Autodesk Inventor part; units mm, degrees
ref_plane "Work Plane8" through (0, 0, 0) normal (0, 0, -1) x (-0.8661856, 0.4997225, 0)
ref_plane "YZ Plane" through (0, 0, 0) normal (1, 0, 0) x (0, 1, 0)
ref_plane "XZ Plane" through (0, 0, 0) normal (0, 1, 0) x (-1, 0, 0)
sketch "Sketch1" plane through (0, 0, 0) normal (0, 0, 1) x (1, 0, 0)
  circle A0 centre (0, 0) radius 14.2875
  circle A1 centre (0, 0) radius 17.4625
  circle A2 centre (0, 0) radius 19.05
  dimension "d0" = 28.575
  dimension "d1" = 34.925
  dimension "d2" = 38.1
extrude "Extrusion1" add sketch "Sketch1" along normal blind 38.1 contours A0 | A1 | A2
sketch "Sketch11" plane through (0, 0, 0) normal (0, 0, 1) x (1, 0, 0)
  circle A0 centre (0, 0) radius 25.908
  circle A1 centre (-38.1, -66.04) radius 12.7
  circle A2 centre (-38.1, -66.04) radius 14.732
  circle A3 centre (-38.1, -66.04) radius 15.748
  line L0 (-38.1, -66.04) -> (-49.1429, -85.181)
  line L1 (-38.1, -66.04) -> (0, 0)
  line L2 (-38.1, -66.04) -> (-49.1551, -46.9061)
  line L3 (-38.1, -66.04) -> (-16.002, -66.0329)
  circle A4 centre (-49.1429, -85.181) radius 1.9844
  circle A5 centre (-49.1551, -46.9061) radius 1.9844
  circle A6 centre (-16.002, -66.0329) radius 1.9844
  circle A7 centre (-16.002, -66.0329) radius 5.5563
  circle A8 centre (-49.1429, -85.181) radius 5.5563
  circle A9 centre (-49.1551, -46.9061) radius 5.5563
  line L4 (-54.6991, -85.1827) -> (-54.7114, -46.9079)
  line L5 (-46.3632, -89.9919) -> (-13.2223, -70.8439)
  line L6 (-13.2254, -61.2202) -> (-46.3785, -42.0934)
  line L7 (0, 0) -> (0, -25.908)
  circle A10 centre (16.002, -66.0329) radius 1.9844
  circle A11 centre (49.1551, -46.9061) radius 1.9844
  circle A12 centre (49.1429, -85.181) radius 1.9844
  line L8 (0, 0) -> (-41.3682, 23.8663)
  line L9 (0, 0) -> (24.0327, 41.6566)
  line L10 (0, 0) -> (61.3648, -35.4028)
  dimension "d137" = 51.816
  dimension "d154" = 0
  dimension "d155" = 360
  dimension "d138" = 38.1
  dimension "d139" = 66.04
  dimension "d140" = 25.4
  dimension "d141" = 29.464
  dimension "d142" = 31.496
  dimension "d143" = 22.098
  dimension "d144" = 120
  dimension "d145" = 120
  dimension "d146" = 22.098
  dimension "d147" = 22.098
  dimension "d148" = 3.9688
  dimension "d149" = 3.9688
  dimension "d150" = 3.9688
  dimension "d151" = 11.1125
  dimension "d152" = 11.1125
  dimension "d153" = 11.1125
  dimension "d159" = 90
  dimension "d160" = 90
  dimension "d161" = 180
ref_plane "Work Plane8" through (0, 0, 0) normal (0, 0, -1) x (-0.8661856, 0.4997225, 0)
sketch "Sketch12" plane through (0, 0, 0) normal (0, 0, -1) x (-0.8661856, 0.4997225, 0)
  circle A0 centre (0, 0) radius 25.908
  circle A1 centre (-38.1, -66.04) radius 12.7
  circle A2 centre (-38.1, -66.04) radius 14.732
  circle A3 centre (-38.1, -66.04) radius 15.748
  line L0 (-38.1, -66.04) -> (-49.1429, -85.181)
  line L1 (-38.1, -66.04) -> (0, 0)
  line L2 (-38.1, -66.04) -> (-49.1551, -46.9061)
  line L3 (-38.1, -66.04) -> (-16.002, -66.0329)
  circle A4 centre (-49.1429, -85.181) radius 1.9844
  circle A5 centre (-49.1551, -46.9061) radius 1.9844
  circle A6 centre (-16.002, -66.0329) radius 1.9844
  circle A7 centre (-16.002, -66.0329) radius 5.5563
  circle A8 centre (-49.1429, -85.181) radius 5.5563
  circle A9 centre (-49.1551, -46.9061) radius 5.5563
  line L4 (-54.6991, -85.1827) -> (-54.7114, -46.9079)
  line L5 (-46.3632, -89.9919) -> (-13.2223, -70.8439)
  line L6 (-13.2254, -61.2202) -> (-46.3785, -42.0934)
  line L7 (0, 0) -> (0, -25.908)
  circle A10 centre (16.002, -66.0329) radius 1.9844
  circle A11 centre (49.1551, -46.9061) radius 1.9844
  circle A12 centre (49.1429, -85.181) radius 1.9844
  dimension "d162" = 51.816
  dimension "d179" = 0
  dimension "d180" = 360
  dimension "d163" = 38.1
  dimension "d164" = 66.04
  dimension "d165" = 25.4
  dimension "d166" = 29.464
  dimension "d167" = 31.496
  dimension "d168" = 22.098
  dimension "d169" = 120
  dimension "d170" = 120
  dimension "d171" = 22.098
  dimension "d172" = 22.098
  dimension "d173" = 3.9688
  dimension "d174" = 3.9688
  dimension "d175" = 3.9688
  dimension "d176" = 11.1125
  dimension "d177" = 11.1125
  dimension "d178" = 11.1125
sketch "Sketch13" plane through (0, 0, 0) normal (0, 1, 0) x (-1, 0, 0)
  line L0 (0, 0) -> (0, 19.05)
  circle A0 centre (0, 19.05) radius 14.2875
  circle A1 centre (0, 19.05) radius 12.7
  dimension "d184" = 19.05
  dimension "d185" = 28.575
  dimension "d186" = 25.4
extrude "Extrusion4" add sketch "Sketch13" against normal blind 25.4 contours A0 | A1
shell "Shell1" thickness 1.5875 removed faces 3 at (-5.6226, 0.0883, 38.1) at (-5.6226, 0.0883, 0) at (-3.9719, -25.4, 19.2449)
extrude "Extrusion5" add sketch "Sketch1" along normal blind 3.175 contours A1
sketch "Sketch14" plane through (0, 0, 38.1) normal (0, 0, 1) x (1, 0, 0)
  circle A0 centre (0, 0) radius 14.2875
  circle A1 centre (0, 0) radius 17.4625
  circle A2 centre (0, 0) radius 19.05
  dimension "d192" = 28.575
  dimension "d193" = 34.925
  dimension "d194" = 38.1
extrude "Extrusion6" add sketch "Sketch14" against normal blind 3.175 contours A1
sketch "Sketch15" plane through (0, -25.4, 19.05) normal (0, -1, 0) x (1, 0, 0)
  circle A0 centre (0, 0) radius 12.7
  circle A1 centre (0, 0) radius 14.2875
  point P0 (0, -19.05)
  dimension "d199" = 25.4
  dimension "d200" = 28.575
sketch3d "3D Sketch4"
  line L0 (0, -25.4, 19.05) -> (0, -57.1923, 19.05)
  arc A0 (0, -57.1923, 19.05) -> (0, -76.2423, 0) centre (0, -57.1923, 0) ccw
  dimension "d198" = 19.05
sweep "Sweep1" add profiles "Sketch15" path "3D Sketch4"
extrude "Extrusion7" add sketch "Sketch12" along normal blind 6.35 contours A1 L3 A2 L0 | A1 L1 A2 L3 | L0 A2 L2 A1 | A1 L2 A2 L1 | L3 A3 L0 A2 | A2 L1 A3 L3 | L0 A3 L2 A2 | A2 L2 A3 L1 | L3 A7 L5 A8 L0 A3 | A3 L1 L6 A7 L3 | L0 A8 L4 A9 L2 A3 | A3 L2 A9 L6 L1 | A7 | A8 | A9
extrude "Extrusion8" add sketch "Sketch12" along normal blind 7.366 contours L3 A3 L0 A2 | A2 L1 A3 L3 | L0 A3 L2 A2 | A2 L2 A3 L1
equation "\"d3\" = 0.9525 * scale"
equation "\"d140\" = 0.635 * d156"
equation "\"d165\" = 0.635 * d181"
equation "\"d36\" = 3.175"
equation "\"d59\" = 3.175"
equation "\"d82\" = 3.175"
equation "\"d104\" = 3.175"
equation "\"d127\" = 3.175"
equation "\"d158\" = 3.175"
equation "\"d183\" = 3.175"
properties part number "Intake_Manifold_2" material "Aluminum 6061"
CAD build for the part. Positions are in the model's coordinates, mm. A direction names the side the tool comes from. Coordinates: 2 decimals unless noted, no trailing zeros. Use CSV: the item, a comma, the result in double quotes. Start each with the question number.
Q1. 3-axis set-ups, long thin cutter, end or side, ignore diameter. For faces 4 (the cylindrical face through (-4, 17, 19)), 5 (the cylindrical face through (23.99, -62.49, -3.13)), 6 (the flat face through (0, -59.637, -3)), 7 (the cylindrical face through (-7.731, -66.167, -3.131)): which of +Z, -Z, +X, -X, +Y, -Y reach the whole face in a straight line?
Q2. Probe probe 1 along Z at (x, y) = (-6, -14.5) (3 decimals); probe 2 along Y at (x, z) = (0, 1.15); probe 3 along Y at (x, z) = (0, 13). List the from-to ranges inside material, lowest first. Write a range as from..to.
Q3. Drop flat-ended pins along their axis: P1, Ø20.5, axis at x = 0, y = -76.24, coming from the -Z side; P2, Ø5, axis at x = 0, y = -98.34, coming from the -Z side; P3, Ø6.5, axis at x = 19.14, y = -65.19, coming from the +Z side; P4, Ø17.5, axis at x = 1, y = 3, coming from the +Z side. Give the stop position or say it passes through.
Q4. Cut at C-C, the plane x = 0. State how many separate pieces and enclosed holes the cut face has, then the cut area to 3 significant figures.
Q5. Two-plate mould, pull along Y, no slides. Class faces 1 (the cylindrical face through (-23.908, -62.345, -3.131)), 2 (the flat face through (-7, -13, 34.925)), 3 (the cylindrical face through (-0.081, -103.896, -3.131)): +Y half, -Y half, draft (parallel to the pull), parting line (faces both ways), or undercut.
Here are the results:
1,face 4,"none"
1,face 5,"+Z, -Z, +X"
1,face 6,"-Z, +X, -X, +Y"
1,face 7,"-Z"
2,probe 1,"0..3.175, 34.925..38.1"
2,probe 2,"-90.51..-88.92, -63.44..-61.81, -19.05..-14.29, 14.29..19.05"
2,probe 3,"-87.89..-86.16, 17.46..19.05"
3,P1,"z = 12.24"
3,P2,"z = -6.35"
3,P3,"z = 0"
3,P4,"through"
4,separate pieces,"4"
4,enclosed holes,"0"
4,area,"434 mm2"
5,face 1,"parting line"
5,face 2,"undercut"
5,face 3,"-Y half"
